from build123d import *
from OCP.BRepFilletAPI import BRepFilletAPI_MakeChamfer

# Parameters (mm, degrees)
BOSS_EXTRUDE1_DEPTH = 11
SKETCH2_W           = 13.6
SKETCH2_H           = 1.1
BOSS_EXTRUDE2_DEPTH = 11
BOSS_EXTRUDE3_DEPTH = 11
SKETCH4_W           = 13.6
SKETCH4_H           = 1.1
BOSS_EXTRUDE4_DEPTH = 11
SKETCH5_W           = 13.6
SKETCH5_H           = 1.1
BOSS_EXTRUDE5_DEPTH = 11
HOLE_WIZARD_M4_1_D  = 4.8
CHAMFER1_SIZE       = 0.85
CHAMFER1_SIZE2      = 1.472243186


with BuildPart() as part:
    # Sketch1 → Boss-Extrude1 (new body)
    with BuildSketch(Plane(origin=(62.103, 0, 0), x_dir=(0, 0, -1), z_dir=(1, 0, 0))):
        with BuildLine():
            Line((34.275005652, 2.916847756), (35.133702257, 4.073392616))
            ThreePointArc((35.133702257, 4.073392616), (40.63247129, 6.846201583), (38.4175, 1.1))
            Line((38.4175, 1.1), (20.4175, 1.1))
            Line((20.4175, 1.1), (20.4175, 0))
            Line((20.4175, 0), (38.4175, 0))
            ThreePointArc((38.4175, 0), (40.950692662, 7.997629072), (34.275005652, 2.916847756))
        make_face()
    extrude(amount=-BOSS_EXTRUDE1_DEPTH)

    # Sketch2 → Boss-Extrude2 (add)
    with BuildSketch(Plane.ZY.offset(-51.103)):
        with Locations((-27.2175, 0.55)):
            Rectangle(SKETCH2_W, SKETCH2_H)
    extrude(amount=BOSS_EXTRUDE2_DEPTH)

    # Sketch3 → Boss-Extrude3 (add)
    with BuildSketch(Plane.ZY.offset(-40.103)):
        with BuildLine():
            Line((-38.4175, 1.1), (-20.4175, 1.1))
            Line((-20.4175, 1.1), (-20.4175, 0))
            Line((-20.4175, 0), (-38.4175, 0))
            ThreePointArc((-38.4175, 0), (-41.043236571, 7.930652555), (-34.203607486, 3.133860244))
            Line((-34.203607486, 3.133860244), (-35.133702257, 4.073392616))
            ThreePointArc((-35.133702257, 4.073392616), (-40.63247129, 6.846201583), (-38.4175, 1.1))
        make_face()
    extrude(amount=BOSS_EXTRUDE3_DEPTH)

    # Sketch4 → Boss-Extrude4 (add)
    with BuildSketch(Plane.ZY.offset(-29.103)):
        with Locations((-27.2175, 0.55)):
            Rectangle(SKETCH4_W, SKETCH4_H)
    extrude(amount=BOSS_EXTRUDE4_DEPTH)

    # Sketch5 → Boss-Extrude5 (add)
    with BuildSketch(Plane(origin=(62.103, 0, 0), x_dir=(0, 0, -1), z_dir=(1, 0, 0))):
        with Locations((27.2175, 0.55)):
            Rectangle(SKETCH5_W, SKETCH5_H)
    extrude(amount=BOSS_EXTRUDE5_DEPTH)

    # M4 间隙孔1 (through all)
    with Locations(Plane(origin=(0, 1.1, 0), x_dir=(1, 0, 0), z_dir=(0, 1, 0))):
        with Locations((45.603, 26.1675), (25.103, 27.1675), (66.103, 27.1675)):
            Hole(HOLE_WIZARD_M4_1_D / 2)

    # Chamfer1: one chamfer whose edges measure the first distance from different faces: ONE call of the kernel's chamfer builder (chamfer() names one face for all edges)
    chamfer1_edges_1 = [part.edges().sort_by_distance(p)[0] for p in [
        (68.503, 0, -27.1675),
    ]]
    chamfer1_side_1 = [part.faces().sort_by_distance(p)[0] for p in [
        (68.503, 0.55, -27.1675),
    ]]
    chamfer1_edges_2 = [part.edges().sort_by_distance(p)[0] for p in [
        (27.503, 0, -27.1675),
    ]]
    chamfer1_side_2 = [part.faces().sort_by_distance(p)[0] for p in [
        (27.503, 0.55, -27.1675),
    ]]
    chamfer1_edges_3 = [part.edges().sort_by_distance(p)[0] for p in [
        (48.003, 0, -26.1675),
    ]]
    chamfer1_side_3 = [part.faces().sort_by_distance(p)[0] for p in [
        (48.003, 0.55, -26.1675),
    ]]
    chamfer1 = BRepFilletAPI_MakeChamfer(part.part.solid().wrapped)
    for e in chamfer1_edges_1:
        chamfer1.Add(CHAMFER1_SIZE, CHAMFER1_SIZE2, e.wrapped, chamfer1_side_1[0].wrapped)  # the first distance lies on this face
    for e in chamfer1_edges_2:
        chamfer1.Add(CHAMFER1_SIZE, CHAMFER1_SIZE2, e.wrapped, chamfer1_side_2[0].wrapped)  # the first distance lies on this face
    for e in chamfer1_edges_3:
        chamfer1.Add(CHAMFER1_SIZE, CHAMFER1_SIZE2, e.wrapped, chamfer1_side_3[0].wrapped)  # the first distance lies on this face
    add(Compound.cast(chamfer1.Shape()), mode=Mode.REPLACE)


solid = part.part
Verification items for the finished model (mm, model axes). A direction names the side the tool comes from. Coordinates: 2 decimals unless noted, no trailing zeros. Write each loop counter-clockwise with the first axis right and the second up, starting at its lowest first coordinate (ties: lowest second). Pieces come first, ordered by that corner, then holes. Notation, with made-up numbers: (-40, 77) -> (17, 77) arc R20 cw to (17, 109) -> close; hole circle Ø2 at (-9.75, 74). An arc over 180 degrees is marked (long way). One line per item, written item: value. Start each with the question number.
Q1. Access from +Z, -Z, +X, -X, +Y, -Y to the whole of each face (thin tool, end or side, straight path). Record for faces 5 (the flat face through (34.68, 3.597, -34.662)), 6 (the flat face through (67.5, 0.5, -34.018)), 7 (the flat face through (51.103, 5, -42)), 8 (the flat face through (29.103, 5, -42)), 9 (the flat face through (56.68, 3.49, -34.7)).
Q2. Go/stop test with flat-tipped pins: P1, Ø5.5, axis at x = 36, z = -26.5, coming from the +Y side; P2, Ø4.5, axis at y = 4.5, z = -37, coming from the -X side; P3, Ø6, axis at x = 66.1, z = -27.17, coming from the -Y side. Record where each tip stops, or that it passes through.
Q3. Cross-section at A-A on y = 5.5. Enter the section's corners in (x, z).
Q4. Cross-section at D-D on z = -33. Enter the section's corners in (x, y), and give its area (3 significant figures).
Q5. Cross-section at C-C on x = 36.5. Enter the section's corners in (y, z), and give its area (3 significant figures).
Q6. Mould release check, pull along X, two halves, no side actions. Record for faces 1 (the flat face through (45.7, 0.5, -34.018)), 2 (the flat face through (18.103, 0.6, -27.3)), 3 (the cylindrical face through (34.68, 6.92, -40.55)), 4 (the flat face through (40.103, 5, -42)): pulls with the +X half, pulls with the -X half, needs draft (parallel to the pull), parting line crosses it, or undercut.
Q7. Thickness scan on L1, parallel to X at y = 8.25, z = -39.75; L2, parallel to Z at x = 58.75, y = 4.4; L3, parallel to Y at x = 36, z = -31.5. Record the ranges inside material, lowest first. Write a range as from..to.
Q8. Cross-section at B-B on y = 2. Enter the section's corners in (x, z), and give its area (3 significant figures).
Checked values:
1. face 5: -X
1. face 6: -Z, +X, +Y, -Y
1. face 7: -Z, +Y, -Y
1. face 8: -Z, -X, +Y, -Y
1. face 9: +X, -X
2. P1: stops at y = 1.1
2. P2: stops at x = 29.1
2. P3: stops at y = 0.5
3. outline: (29.1, -42.68) -> (40.1, -42.68) -> (40.1, -41.53) -> (29.1, -41.53) -> close; (29.1, -35.31) -> (40.1, -35.31) -> (40.1, -34.16) -> (29.1, -34.16) -> close; (51.1, -42.68) -> (62.1, -42.68) -> (62.1, -41.53) -> (51.1, -41.53) -> close; (51.1, -35.31) -> (62.1, -35.31) -> (62.1, -34.16) -> (51.1, -34.16) -> close
4. outline: (18.1, 0) -> (73.1, 0) -> (73.1, 1.1) -> (18.1, 1.1) -> close
4. area: 60.5 mm²
5. outline: (0, -38.42) arc R4.4 ccw (long way) to (3.13, -34.2) -> (4.07, -35.13) arc R3.3 cw (long way) to (1.1, -38.42) -> (1.1, -20.42) -> (0, -20.42) -> close
5. area: 40.7 mm²
6. face 1: undercut
6. face 2: pulls with the -X half
6. face 3: needs draft
6. face 4: undercut
7. L1: x = 29.1..40.1, 51.1..62.1
7. L2: z = -42.82..-41.72, -35.12..-34.02
7. L3: y = 0..1.1
8. outline: (29.1, -42.11) -> (40.1, -42.11) -> (40.1, -40.68) -> (29.1, -40.68) -> close; (51.1, -42.11) -> (62.1, -42.11) -> (62.1, -40.68) -> (51.1, -40.68) -> close
8. area: 31.3 mm²
